Solid Edge part; units mm, degrees
sketch "Sketch1" plane through (0, 0, 0) normal (0, -1, 0) x (1, 0, 0)
  line L0 (3.13, 1) -> (1.35, 1)
  line L1 (1.35, 1) -> (1.35, 2.5)
  line L2 (1.35, 2.5) -> (2, 2.5)
  line L3 (2, 2.5) -> (2, 3)
  line L4 (1.35, 3) -> (2, 3)
  line L5 (1.35, 5) -> (1.35, 3)
  line L6 (1.35, 5) -> (1.25, 5)
  line L7 (1.25, 5) -> (1.25, 0)
  line L8 (1.25, 0) -> (3.13, 0)
  line L9 (3.13, 0) -> (3.13, 1)
revolve "RevolvedProtrusion1" add sketch "Sketch1" angle 360 about axis through (0, 0, 5) along (0, 0, -1)
properties material "Galvanized steel"
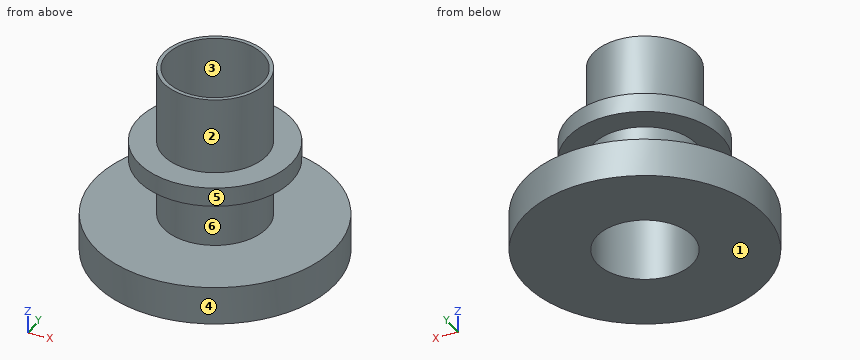
Input: part model. Units: mm. Frame: model coordinates. Face numbers are marked on the shaded views. A direction names the side the tool comes from. Coordinates: 2 decimals unless noted, no trailing zeros. Loops run counter-clockwise (first coordinate to the right, second up) from the corner with the lowest first, then second, coordinate; pieces in that order, holes last. Notation, with made-up numbers: M 80.5,2 L 128.5,2 A18 ccw 128.5,27 Z; hole C -17.75,-1 d10. An arc over 180 degrees is marked long. Use a Markdown table: item, result. Add a question column.
1) Section D-D, the plane x = 1.75. Return the cut outline in (y, z), plus the area to 3 significant figures.
2) Section C-C, the plane z = 3.75. Return the cut outline in (x, y).
3) Pin query (flat end, axial travel): P1, Ø2, axis at y = 0, z = 3.5, coming from the +X side; P2, Ø2, axis at x = 0, y = 0, coming from the -Z side. Return the tip coordinate at first contact, or that it passes through.
4) Draft query along Y for the marked faces 1, 2 and 3. Return one class per face: +Y half, -Y half, draft (parallel to the pull), parting line (faces both ways), or undercut.
5) Set-up query: the marked faces 4, 5 and 6. Return all of +Z, -Z, +X, -X, +Y, -Y with unobstructed straight access to the full face (end or side cutting, diameter ignored); none if empty.
6) Section A-A, the plane y = 0. Return the cut outline in (x, z), plus the area to 3 significant figures.
7) Line query: L1, parallel to Z at x = -1.5, y = 0; L2, parallel to Z at x = 1.5, y = -2.25; L3, parallel to X at y = 0, z = 2.9. Output: solid intervals per line, ascending. Write a range as from..to.
Answer below:
| question | item | result |
|---|---|---|
| 1 | outline | M -2.6,0 L 2.6,0 L 2.6,1 L -2.6,1 Z; M -0.97,2.5 L 0.97,2.5 L 0.97,3 L -0.97,3 Z |
| 1 | area | 6.16 mm2 |
| 2 | outline | C 0,0 d2.7; hole C 0,0 d2.5 |
| 3 | P1 | x = 2 |
| 3 | P2 | through |
| 4 | face 1 | draft |
| 4 | face 2 | parting line |
| 4 | face 3 | undercut |
| 5 | face 4 | +Z, -Z |
| 5 | face 5 | +Z |
| 5 | face 6 | none |
| 6 | outline | M -3.13,0 L -1.25,0 L -1.25,5 L -1.35,5 L -1.35,3 L -2,3 L -2,2.5 L -1.35,2.5 L -1.35,1 L -3.13,1 Z; M 1.25,0 L 3.13,0 L 3.13,1 L 1.35,1 L 1.35,2.5 L 2,2.5 L 2,3 L 1.35,3 L 1.35,5 L 1.25,5 Z |
| 6 | area | 5.21 mm2 |
| 7 | L1 | 0..1, 2.5..3 |
| 7 | L2 | 0..1 |
| 7 | L3 | -2..-1.25, 1.25..2 |
